```python
from build123d import *

# Parameters (mm, degrees)
F1_DEPTH = 28
F3_DEPTH = 94
F5_DEPTH = 28
F6_R     = 2
F7_R     = 1
F8_R     = 4.25
F9_DEPTH = 25


with BuildPart() as f1:
    # F0 (on Top) → F1 (new body)
    with BuildSketch(Plane.XY):
        Polygon((-19.75, -17.750001), (-19.75, -19.75), (-9.25, -19.75), (19.75, 9.25), (19.75, 19.75), (17.750001, 19.75), (17.750001, 10.078427), (-10.078427, -17.750001), align=None)
    extrude(amount=F1_DEPTH)

    # F2 (on face) → F3 (join)
    with BuildSketch(Plane.XY.offset(28)):
        Polygon((-19.75, -19.75), (-9.25, -19.75), (19.75, 9.25), (19.75, 19.75), (11.25, 19.75), (11.25, 24.25), (9.25, 26.25), (9.25, 23.421573), (9.25, 19.75), (9.25, 17.750001), (17.750001, 17.750001), (17.750001, 10.078427), (16.585787, 8.914213), (-8.914213, -16.585787), (-10.078427, -17.750001), (-17.750001, -17.750001), (-17.750001, -9.25), (-19.75, -9.25), (-23.421573, -9.25), (-26.25, -9.25), (-24.25, -11.25), (-19.75, -11.25), align=None)
    extrude(amount=F3_DEPTH)

    # F4 (on face) → F5 (join)
    with BuildSketch(Plane.XY.offset(122)):
        Polygon((19.75, 9.25), (19.75, 19.75), (17.750001, 19.75), (17.750001, 10.078427), (-10.078427, -17.750001), (-19.75, -17.750001), (-19.75, -19.75), (-9.25, -19.75), align=None)
    extrude(amount=F5_DEPTH)

    # F6
    f6_edges = [f1.edges().sort_by_distance(p)[0] for p in [
        (19.75, 9.25, 75),
        (-9.25, -19.75, 75),
    ]]
    fillet(f6_edges, radius=F6_R)

    # F7
    f7_edges = [f1.edges().sort_by_distance(p)[0] for p in [
        (-19.75, -19.75, 75),
        (19.75, 19.75, 75),
    ]]
    fillet(f7_edges, radius=F7_R)

    # F8 (on face) → F9 (cut)
    with BuildSketch(Plane(origin=(5.25, -5.25, 0), x_dir=(0.707107, 0.707107, 0), z_dir=(0.707107, -0.707107, 0))):
        with Locations((0, 136)):
            Circle(F8_R)
    extrude(amount=-F9_DEPTH, mode=Mode.SUBTRACT)


solid = f1.part
```
Work out the finished part from the listing and answer in its coordinate system (mm). A direction names the side the tool comes from. Round coordinates to 2 decimals unless told otherwise and drop trailing zeros. Write each loop counter-clockwise with the first axis right and the second up, starting at its lowest first coordinate (ties: lowest second). Pieces come first, ordered by that corner, then holes. Notation, with made-up numbers: (-7.75, 43) - (43.25, 43) arc R9 cw to (43.25, 55) - close; hole circle Ø3 at (-38, 52.25). An arc over 180 degrees is marked (long way). Return JSON: item names as keys, results as strings. Group by question number.
Q1. Each of these flat-tipped pins is pushed along its axis until it touches: pin 1 Ø7 at (x, y) = (15, 20.5) entering from +Z; pin 2 Ø1.5 at (x, z) = (-1.5, 42) entering from -Y; pin 3 Ø1.3 at (y, z) = (23, 96.5) entering from +X; pin 4 Ø6 at (x, z) = (16.5, 107.5) entering from +Y. Where does it stop, or does it pass through?
Q2. The part is cut by section A-A on z = 124.5. Write down the section's boundary in (x, y).
Q3. The part is cut by section D-D on y = 15.5. Write down the section's boundary in (x, z).
Q4. The mould has two halves that part along X. Classify faces 6 (the flat face through (9.25, 22, 74)), 7 (the flat face through (-19.5, -12.2, 122)), 8 (the flat face through (-15, -17.75, 74)), 9 (the flat face through (-17.75, -14, 74)): released by +X, released by -X, zero draft, split by the parting line, or undercut.
Q5. Find the intervals of material crossed by L1, parallel to X at y = 13, z = 41.5; L2, parallel to X at y = -9.5, z = 96; L3, parallel to Y at x = 11, z = 102, in increasing order.
Q6. The part is cut by section B-B on x = -15.5. Write down the section's boundary in (y, z), then the cut area to 3 significant figures.
Q7. The part is cut by section C-C on z = 32. Write down the section's boundary in (x, y), then the cut area to 3 significant figures.
Q8. For faces 1 (the flat face through (11.25, 22, 74)), 2 (the flat face through (13, 17.75, 74)), 3 (the flat face through (-22, -9.25, 74)), 4 (the flat face through (-19.75, -15, 74)), 5 (the flat face through (12.2, 19.5, 122)), determine the directions among +Z, -Z, +X, -X, +Y, -Y from which every point of the face is accessible in a straight line to the end or side of a thin tool.
Solved:
{
 "1": {"pin 1": "z = 150", "pin 2": "y = -12.75", "pin 3": "x = 11.25", "pin 4": "y = 19.75"},
 "2": {"outline": "(-19.75, -18.75) arc R1 ccw to (-18.75, -19.75) - (-10.08, -19.75) arc R2 ccw to (-8.66, -19.16) - (19.16, 8.66) arc R2 ccw to (19.75, 10.08) - (19.75, 18.75) arc R1 ccw to (18.75, 19.75) - (17.75, 19.75) - (17.75, 10.08) - (-10.08, -17.75) - (-19.75, -17.75) - close"},
 "3": {"outline": "(17.75, 0) - (19.75, 0) - (19.75, 150) - (17.75, 150) - close"},
 "4": {"face 6": "released by -X", "face 7": "zero draft", "face 8": "undercut", "face 9": "undercut"},
 "5": {"L1": "17.75 to 19.75", "L2": "-26 to -17.75, -1.83 to 1", "L3": "0.5 to 3.33, 17.75 to 24.5"},
 "6": {"outline": "(-19.75, 0) - (-17.75, 0) - (-17.75, 150) - (-19.75, 150) - close", "area": "300 mm²"},
 "7": {"outline": "(-26.25, -9.25) - (-24.25, -11.25) - (-19.75, -11.25) - (-19.75, -18.75) arc R1 ccw to (-18.75, -19.75) - (-10.08, -19.75) arc R2 ccw to (-8.66, -19.16) - (19.16, 8.66) arc R2 ccw to (19.75, 10.08) - (19.75, 18.75) arc R1 ccw to (18.75, 19.75) - (11.25, 19.75) - (11.25, 24.25) - (9.25, 26.25) - (9.25, 17.75) - (17.75, 17.75) - (17.75, 10.08) - (-10.08, -17.75) - (-17.75, -17.75) - (-17.75, -9.25) - close", "area": "176 mm²"},
 "8": {"face 1": "+Z, -Z, +X, +Y", "face 2": "+Z, -Z, -X", "face 3": "+Z, -Z, -X, +Y", "face 4": "+Z, -Z, -X, -Y", "face 5": "+Z, -X, +Y"}
}
